Could you check a few things on this model? Use its own coordinates, in mm. A direction names the side the tool comes from. Coordinates: 2 decimals unless noted, no trailing zeros. Loops run counter-clockwise (first coordinate to the right, second up) from the corner with the lowest first, then second, coordinate; pieces in that order, holes last. Notation, with made-up numbers: (61, 76.5) - (103, 76.5) arc R5 cw to (103, 84.5) - close; hole circle Ø7 at (81, -21.5). An arc over 180 degrees is marked (long way). One line per question, with ' | ' between items. Start each with the question number.
1. I want a section at B-B, the plane z = 3. Write out the boundary of the cut face in (x, y).
2. Which directions (+Z, -Z, +X, -X, +Y, -Y) give clear straight access to the entire face, cutting with the end or side of a thin tool? Please do faces 1 (the flat face through (17, 3, 0)), 2 (the flat face through (0, 2, 0)).
3. I want a section at C-C, the plane x = 8.5. Write out the boundary of the cut face in (y, z).
4. Please list where these lines run through material, in increasing order: L1, parallel to X at y = 4.5, z = -1; L2, parallel to Y at x = 13, z = 5. Write a range as [from, to].
5. I'm going to push a flat-ended pin straight in: P1, Ø9, axis at x = 0.5, z = -0.5, coming from the +Y side. Where does the tip first touch, or does it pass through?
6. I want a section at A-A, the plane y = 2.75. Write out the boundary of the cut face in (x, z).
7. I want a section at D-D, the plane x = -2.5. Write out the boundary of the cut face in (y, z), then the cut area to 3 significant figures.
8. We'd pull the mould along Z, two halves only. Please class faces 3 (the flat face through (0, 8, -16)), 4 (the cylindrical face through (-0.12, 7.49, -16.89)), 5 (the cylindrical face through (14.57, 4.54, -14.55)): pulls with the +Z half, pulls with the -Z half, needs draft (parallel to the pull), parting line crosses it, or undercut.
from build123d import *

# Parameters (mm, degrees)
SKETCH1_W           = 30
SKETCH1_H           = 30
BOSS_EXTRUDE2_DEPTH = 2
SKETCH1_6_W         = 34
SKETCH1_6_H         = 34
SKETCH1_6_W_2       = 30
SKETCH1_6_H_2       = 30
BOSS_EXTRUDE3_DEPTH = 7
FILLET1_R           = 1.5
SKETCH2_R           = 0.9
BOSS_EXTRUDE4_DEPTH = 1


with BuildPart() as part:
    # Sketch1 → Boss-Extrude2 (new body)
    with BuildSketch(Plane(origin=(0, 0, 0), x_dir=(1, 0, 0), z_dir=(0, 1, 0))):
        Rectangle(SKETCH1_W, SKETCH1_H)
    extrude(amount=BOSS_EXTRUDE2_DEPTH)

    # Sketch1<6> → Boss-Extrude3 (add)
    with BuildSketch(Plane(origin=(0, 0, 0), x_dir=(1, 0, 0), z_dir=(0, 1, 0))):
        Rectangle(SKETCH1_6_W, SKETCH1_6_H)
        Rectangle(SKETCH1_6_W_2, SKETCH1_6_H_2, mode=Mode.SUBTRACT)
    extrude(amount=BOSS_EXTRUDE3_DEPTH)

    # Fillet1
    fillet1_edges = [part.edges().sort_by_distance(p)[0] for p in [
        (15, 4.5, -15),
        (-15, 4.5, -15),
        (-15, 4.5, 15),
        (15, 4.5, 15),
    ]]
    fillet(fillet1_edges, radius=FILLET1_R)

    # Sketch2 → Boss-Extrude4 (add)
    with BuildSketch(Plane(origin=(0, 7, 0), x_dir=(1, 0, 0), z_dir=(0, 1, 0))):
        with Locations((0, 16)):
            Circle(SKETCH2_R)
        with Locations((-2.5, 16)):
            Circle(SKETCH2_R)
        with Locations((-5, 16)):
            Circle(SKETCH2_R)
        with Locations((2.5, 16)):
            Circle(SKETCH2_R)
        with Locations((5, 16)):
            Circle(SKETCH2_R)
    extrude(amount=BOSS_EXTRUDE4_DEPTH)


solid = part.part
Results are:
1) outline: (-17, 0) - (17, 0) - (17, 7) - (15, 7) - (15, 2) - (-15, 2) - (-15, 7) - (-17, 7) - close
2) face 1: +Z, -Z, +X, +Y, -Y | face 2: +Y
3) outline: (0, -17) - (7, -17) - (7, -15) - (2, -15) - (2, 15) - (7, 15) - (7, 17) - (0, 17) - close
4) L1: x = [-17, -15], [15, 17] | L2: y = [0, 2]
5) P1: stops at y = 2
6) outline: (-17, -17) - (17, -17) - (17, 17) - (-17, 17) - close; hole (-15, -13.5) arc R1.5 ccw to (-13.5, -15) - (13.5, -15) arc R1.5 ccw to (15, -13.5) - (15, 13.5) arc R1.5 ccw to (13.5, 15) - (-13.5, 15) arc R1.5 ccw to (-15, 13.5) - close
7) outline: (0, -17) - (7, -17) - (7, -16.9) - (8, -16.9) - (8, -15.1) - (7, -15.1) - (7, -15) - (2, -15) - (2, 15) - (7, 15) - (7, 17) - (0, 17) - close | area: 89.8 mm2
8) face 3: needs draft | face 4: parting line crosses it | face 5: undercut
